The drawing under review shows one solid part. Ordinate dimensions are in mm from its lowest x, y, z. A direction names the side the tool comes from. Give positions to 0.01 mm unless a question says otherwise; leave off trailing zeros. Write each loop counter-clockwise with the first axis right and the second up, starting at its lowest first coordinate (ties: lowest second). Pieces come first, ordered by that corner, then holes.
Q1. Machinability: for the marked faces 1, 2 and 3, which of the approach directions +Z, -Z, +X, -X, +Y, -Y give a long, thin tool a straight path to every point of the face, cutting with its end or side? Answer none if there is none.
Q2. Mouldability with a two-part tool opening along Y and no side actions: class the marked faces 4, 5 and 6 as released by +Y, released by -Y, zero draft, split by the parting line, or undercut.
Q3. We need section D-D (x = 14). Write out the cut boundary in (y, z).
Q4. Insertion check: P1, Ø11, axis at x = 23, y = 26, coming from the +Z side; P2, Ø10, axis at y = 44, z = 6.5, coming from the -X side; P3, Ø8, axis at x = 25.5, y = 26, coming from the -Z side; P4, Ø10, axis at x = 26.5, y = 40, coming from the -Z side. Each pin has a flat end and moves straight along its axis. Give the tip position at first contact, or say it passes through.
Q5. For line 1 (Y direction, x = 25, z = 2); line 2 (Z direction, x = 28, y = 8.5); line 3 (X direction, y = 8.5, z = 7), list the stretches that pass through material, from the lowest coordinate up.
Q6. We need section A-A (y = 25). Write out the cut boundary in (x, z) (3 decimals).
Q7. We need section C-C (z = 4.25). Write out the cut boundary in (x, y), then the cut area to 3 significant figures.
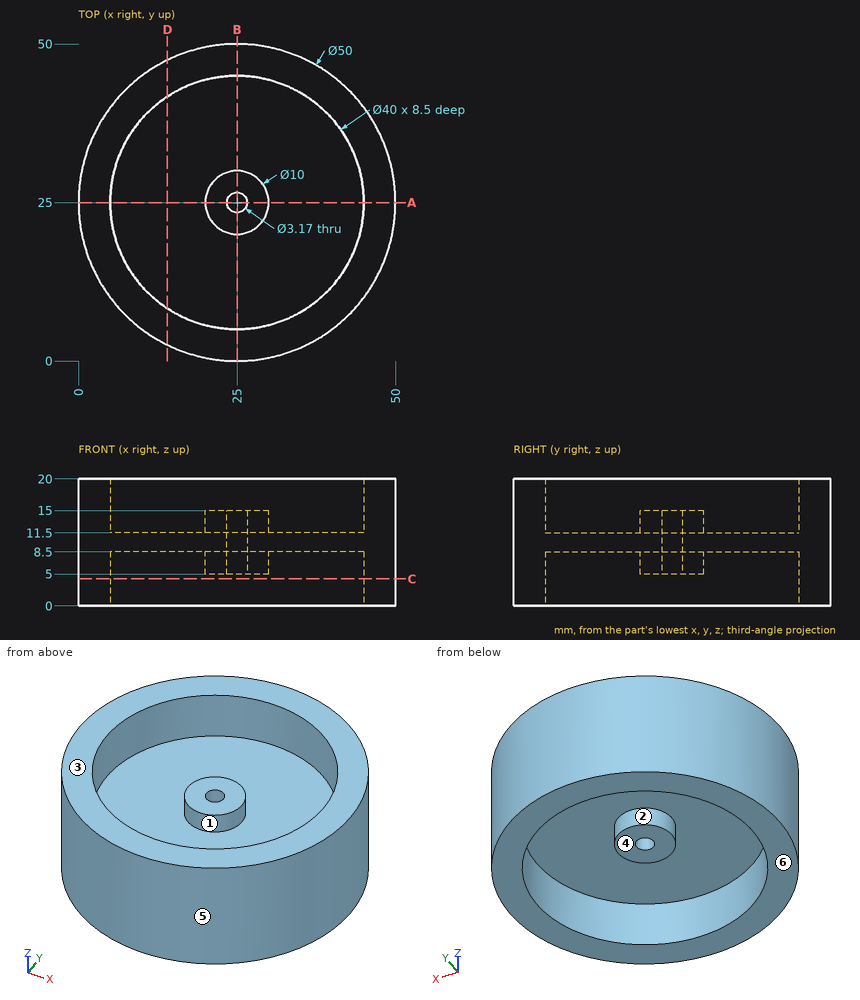
Computed:
1. face 1: +Z
1. face 2: -Z
1. face 3: +Z, +X, -X, +Y, -Y
2. face 4: undercut
2. face 5: split by the parting line
2. face 6: zero draft
3. outline: (2.55, 0) - (8.3, 0) - (8.3, 8.5) - (41.7, 8.5) - (41.7, 0) - (47.45, 0) - (47.45, 20) - (41.7, 20) - (41.7, 11.5) - (8.3, 11.5) - (8.3, 20) - (2.55, 20) - close
4. P1: stops at z = 15
4. P2: stops at x = 4.29
4. P3: stops at z = 5
4. P4: stops at z = 0
5. line 1: y = 0 to 5, 45 to 50
5. line 2: z = 8.5 to 11.5
5. line 3: x = 6.22 to 13.7, 36.3 to 43.78
6. outline: (0, 0) - (5, 0) - (5, 8.5) - (20, 8.5) - (20, 5) - (23.415, 5) - (23.415, 15) - (20, 15) - (20, 11.5) - (5, 11.5) - (5, 20) - (0, 20) - close; (26.585, 5) - (30, 5) - (30, 8.5) - (45, 8.5) - (45, 0) - (50, 0) - (50, 20) - (45, 20) - (45, 11.5) - (30, 11.5) - (30, 15) - (26.585, 15) - close
7. outline: circle Ø50 at (25, 25); hole circle Ø40 at (25, 25)
7. area: 707 mm2
